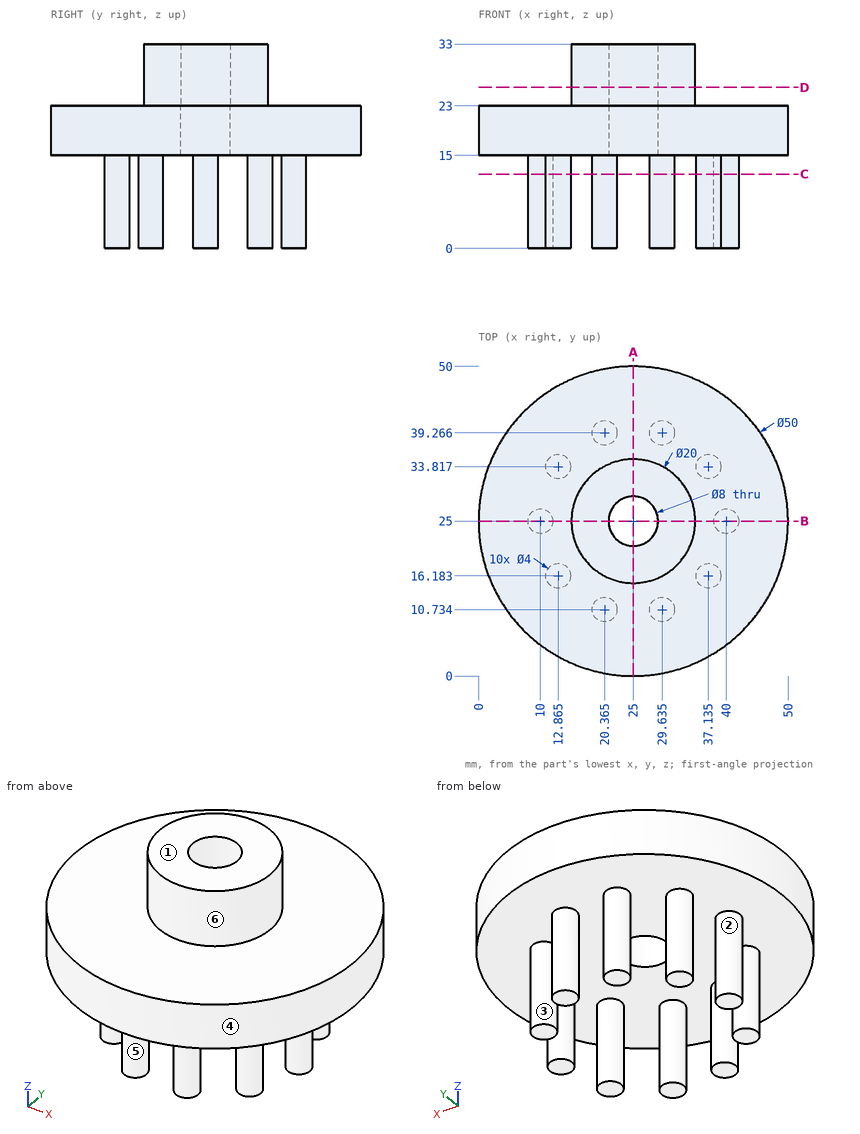
Here's the drawing with two shaded views (mm, measured from the low corner). I have some questions. A direction names the side the tool comes from. Give positions to 0.01 mm unless a question says otherwise; leave off trailing zeros. Loops run counter-clockwise (first coordinate to the right, second up) from the corner with the lowest first, then second, coordinate; pieces in that order, holes last. Notation, with made-up numbers: M -37.75,-2 L -28.75,-2 A32 ccw -28.75,31 Z; hole C -14.75,2.5 d3. An arc over 180 degrees is marked long. Use one line per item in the form item = value. Start each with the question number.
Q1. Thinking about a two-plate mould opening in X: for the marked faces 1, 2, 3 and 4, which applies, +X half, -X half, draft (parallel to the pull), parting line (faces both ways), or undercut?
Q2. I need wall thicknesses on line 1 along Y through (x, z) = (25, 19.25); line 2 along X through (y, z) = (16, 11); line 3 along X through (y, z) = (25, 7.5). Which ranges of each line are inside material? Lowest first, please.
Q3. If we section it at C-C (z = 12): State how many separate pieces and enclosed holes the cut face has, then the cut area to 3 significant figures.
Q4. Which directions (+Z, -Z, +X, -X, +Y, -Y) give clear straight access to the entire face, cutting with the end or side of a thin tool? Please do the marked faces 5 and 6.
Q5. Will these pins go through, and if not, where does the flat tip stop? pin 1 Ø3 at (y, z) = (11, 5.5) entering from -X (1 decimal); pin 2 Ø1 at (x, y) = (28, 42) entering from -Z; pin 3 Ø5 at (x, y) = (25, 25) entering from -Z; pin 4 Ø12 at (x, y) = (41.5, 13.5) entering from +Z.
Q6. If we section it at A-A (x = 25): Write out the boundary of the cut face in (y, z).
Q7. If we section it at B-B (y = 25): Write out the boundary of the cut face in (x, z), then the cut area to 3 significant figures.
Q8. If we section it at D-D (z = 26): Write out the boundary of the cut face in (x, y).
Taken from the geometry:
q1.face_1 = draft
q1.face_2 = undercut
q1.face_3 = undercut
q1.face_4 = parting line
q2.line_1 = 0 to 21, 29 to 50
q2.line_2 = 10.87 to 14.86, 35.14 to 39.13
q2.line_3 = 8 to 12, 38 to 42
q3.separate_pieces = 10
q3.enclosed_holes = 0
q3.area = 126 mm^2
q4.face_5 = -Z
q4.face_6 = +Z
q5.pin_1 = 18.4
q5.pin_2 = 15
q5.pin_3 = through
q5.pin_4 = 23
q6.outline = M 0,15 L 21,15 L 21,33 L 15,33 L 15,23 L 0,23 Z; M 29,15 L 50,15 L 50,23 L 35,23 L 35,33 L 29,33 Z
q7.outline = M 0,15 L 8,15 L 8,0 L 12,0 L 12,15 L 21,15 L 21,33 L 15,33 L 15,23 L 0,23 Z; M 29,15 L 38,15 L 38,0 L 42,0 L 42,15 L 50,15 L 50,23 L 35,23 L 35,33 L 29,33 Z
q7.area = 576 mm^2
q8.outline = C 25,25 d20; hole C 25,25 d8
